from build123d import *

# Parameters (mm, degrees)
F0_W          = 101.6
F0_H          = 25.4
F1_DEPTH      = 3.175
F1_DEPTH_BACK = 3.175
F2_R          = 6.35
F3_DEPTH      = 6.351
F4_DEPTH      = 6.351
F5_R          = 12.69999


# Not quite as in the source:
# - a fillet or chamfer is up to 0.001 mm smaller than in the source, because OpenCascade refuses the exact size


with BuildPart() as f1:
    # F0 (on Top) → F1 (new body, two sides)
    with BuildSketch(Plane.XY) as f1_sk:
        Rectangle(F0_W, F0_H)
    extrude(amount=F1_DEPTH)
    extrude(f1_sk.sketch, amount=-F1_DEPTH_BACK)

    # F2 (on face) → F3 (cut, through all)
    with BuildSketch(Plane.XY.offset(3.175)):
        with Locations((38.1, 0)):
            Circle(F2_R)
        with Locations((-38.1, 0)):
            Circle(F2_R)
    extrude(amount=-F3_DEPTH, mode=Mode.SUBTRACT)

    # F2 (on face) → F4 (cut, through all)
    with BuildSketch(Plane.XY.offset(3.175)):
        with Locations((38.1, 0)):
            Circle(F2_R)
        with Locations((-38.1, 0)):
            Circle(F2_R)
    extrude(amount=-F4_DEPTH, mode=Mode.SUBTRACT)

    # F5 (radius 12.7 in the source; OpenCascade refuses exactly that, so slightly less here)
    f5_edges = [f1.edges().sort_by_distance(p)[0] for p in [
        (50.8, -12.7, 0),
        (-50.8, -12.7, 0),
        (50.8, 12.7, 0),
        (-50.8, 12.7, 0),
    ]]
    fillet(f5_edges, radius=F5_R)


solid = f1.part
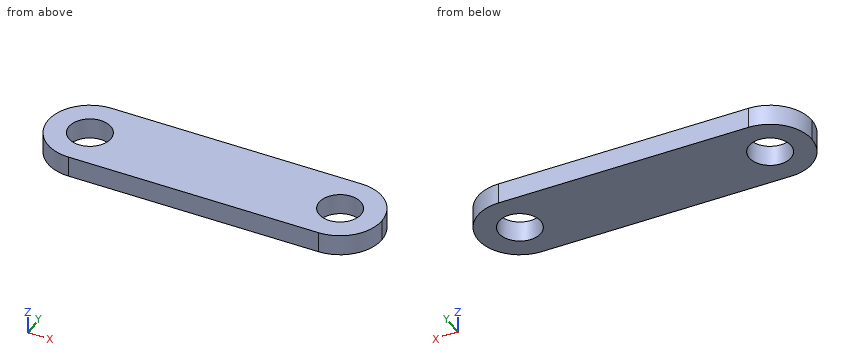
Input: part model. Units: mm. Frame: model coordinates. Give positions to 0.01 mm unless a question says otherwise; leave off trailing zeros. Loops run counter-clockwise (first coordinate to the right, second up) from the corner with the lowest first, then second, coordinate; pieces in that order, holes last. Notation, with made-up numbers: M 13.25,0.5 L 23.25,0.5 A29 cw 23.25,39.5 Z; hole C -28,38.5 d3. An arc over 180 degrees is marked long. Use CSV: the item, a comma, the result in double quotes.
(1) Section A-A, the plane y = 4. Return loops of the section in (x, z) (3 decimals), plus the area to 3 significant figures.
Outcome:
outline,"M -50.154,-3.175 L -43.032,-3.175 L -43.032,3.175 L -50.154,3.175 Z; M -33.168,-3.175 L 33.168,-3.175 L 33.168,3.175 L -33.168,3.175 Z; M 43.032,-3.175 L 50.154,-3.175 L 50.154,3.175 L 43.032,3.175 Z"
area,"512 mm²"
(2) Section B-B, the plane x = 42. Return loops of the section in (y, z) (3 decimals), plus the area to 3 significant figures.
Outcome:
outline,"M -12.086,-3.175 L -5.011,-3.175 L -5.011,3.175 L -12.086,3.175 Z; M 5.011,-3.175 L 12.086,-3.175 L 12.086,3.175 L 5.011,3.175 Z"
area,"89.9 mm²"
(3) Section C-C, the plane z = -0.5. Count the separate pieces of the cut face and the enclosed holes in it, plus the area to 3 significant figures.
Outcome:
separate pieces,"1"
enclosed holes,"2"
area,"2,190 mm²"
(4) Material intervals for L1, parallel to X at y = 4.25, z = -0.75; L2, parallel to Y at x = 38.1, z = -1.5; L3, parallel to X at y = -11, z = -1.25, sorted ascending. Write a range as [from, to].
Outcome:
L1,"x = [-50.07, -42.82], [-33.38, 33.38], [42.82, 50.07]"
L2,"y = [-12.7, -6.35], [6.35, 12.7]"
L3,"x = [-44.45, 44.45]"
(5) Pin query (flat end, axial travel): P1, Ø2, axis at y = 9, z = 1, coming from the -X side; P2, Ø1.5, axis at y = -1.5, z = 2, coming from the -X side. Return the tip coordinate at first contact, or that it passes through.
Outcome:
P1,"stops at x = -47.96"
P2,"stops at x = -50.78"
(6) Section D-D, the plane y = 8.25. Return loops of the section in (x, z) (3 decimals), plus the area to 3 significant figures.
Outcome:
outline,"M -47.755,-3.175 L 47.755,-3.175 L 47.755,3.175 L -47.755,3.175 Z"
area,"606 mm²"
